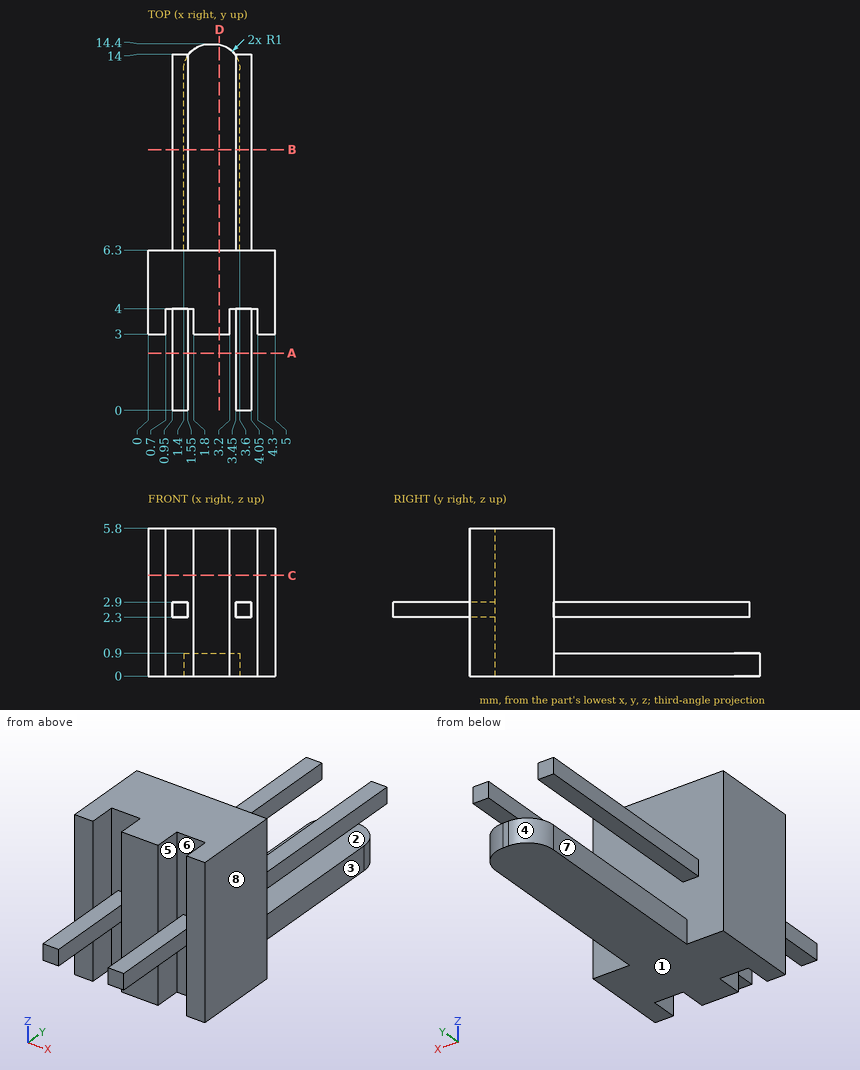
Can you work these out from the drawing? Everything is in mm from the part's minimum corner. A direction names the side the tool comes from. Coordinates: 2 decimals unless noted, no trailing zeros. Order: outer loops, then holes, each group sorted by start corner. A loop starts at its lowest first (then second) coordinate and runs counter-clockwise, first axis right, second up. Notation, with made-up numbers: (65, 32.25) -> (86, 32.25) arc R29 ccw to (86, 54.25) -> close; hole circle Ø6 at (36.5, 14). An arc over 180 degrees is marked (long way). Use one line per item in the form item = value.
Q1. Imagine slicing it at A-A, the plane y = 2.25. List the corners of the cut face in (x, z) for me.
From the geometry:
outline = (0.95, 2.3) -> (1.55, 2.3) -> (1.55, 2.9) -> (0.95, 2.9) -> close; (3.45, 2.3) -> (4.05, 2.3) -> (4.05, 2.9) -> (3.45, 2.9) -> close
Q2. Imagine slicing it at C-C, the plane z = 3.95. List the corners of the cut face in (x, y) for me.
From the geometry:
outline = (0, 3) -> (0.7, 3) -> (0.7, 4) -> (1.8, 4) -> (1.8, 3) -> (3.2, 3) -> (3.2, 4) -> (4.3, 4) -> (4.3, 3) -> (5, 3) -> (5, 6.3) -> (0, 6.3) -> close
Q3. Imagine slicing it at B-B, the plane y = 10.25. List the corners of the cut face in (x, z) for me.
From the geometry:
outline = (0.95, 2.3) -> (1.55, 2.3) -> (1.55, 2.9) -> (0.95, 2.9) -> close; (1.4, 0) -> (3.6, 0) -> (3.6, 0.9) -> (1.4, 0.9) -> close; (3.45, 2.3) -> (4.05, 2.3) -> (4.05, 2.9) -> (3.45, 2.9) -> close
Q4. Will these pins go through, and if not, where does the flat tip stop? P1, Ø1.5, axis at x = 2.5, z = 3, coming from the +Y side; P2, Ø1.5, axis at x = 3.5, y = 9.5, coming from the +Z side; P3, Ø0.5, axis at y = 12, z = 2.5, coming from the +X side.
From the geometry:
P1 = 6.3
P2 = 2.9
P3 = 4.05
Q5. We'd pull the mould along X, two halves only. Please class the marked faces 6, 7 and 8: released by +X, released by -X, zero draft, split by the parting line, or undercut.
From the geometry:
face_6 = undercut
face_7 = released by -X
face_8 = released by +X
Q6. Which directions (+Z, -Z, +X, -X, +Y, -Y) give clear straight access to the entire face, cutting with the end or side of a thin tool? Please do the marked faces 1, 2, 3, 4 and 5.
From the geometry:
face_1 = -Z, +X, -X, +Y, -Y
face_2 = +X, -X, +Y
face_3 = -Z, +X, +Y
face_4 = -Z, -X, +Y
face_5 = +Z, -Z, -Y
Q7. Imagine slicing it at D-D, the plane x = 2.8. List the corners of the cut face in (y, z) for me.
From the geometry:
outline = (3, 0) -> (14.38, 0) -> (14.38, 0.9) -> (6.3, 0.9) -> (6.3, 5.8) -> (3, 5.8) -> close
Q8. I need wall thicknesses on L1, parallel to X at y = 3.75, z = 2.05; L2, parallel to Y at x = 1.05, z = 3.25; L3, parallel to Y at x = 2.95, z = 3.9. Which ranges of each line are inside material? Lowest first, please.
From the geometry:
L1 = 0 to 0.7, 1.8 to 3.2, 4.3 to 5
L2 = 4 to 6.3
L3 = 3 to 6.3
